from build123d import *

# Parameters (mm, degrees)
SKETCH1_R           = 5
BOSS_EXTRUDE1_DEPTH = 5


with BuildPart() as part:
    # Sketch1 → Boss-Extrude1 (new body)
    with BuildSketch(Plane.XY):
        Polygon((-56.800385751, 0), (-54.300385751, 0), (-54.300385751, -5), (-44.300385751, -5), (-44.300385751, 0), (-35.800385751, 0), (-35.800385751, 3), (-36.900385751, 3), (-36.900385751, 5.3), (-35.800385751, 5.3), (-35.800385751, 10), (-32.800385751, 10), (-32.800385751, 5.3), (-31.700385751, 5.3), (-31.700385751, 3), (-32.800385751, 3), (-32.800385751, 0), (-24.300385751, 0), (-24.300385751, -5), (-14.300385751, -5), (-14.300385751, -0.020707798), (-11.800385751, -0.020707798), (-11.800385751, 220), (-14.300385751, 220), (-14.300385751, 225), (-24.300385751, 225), (-24.300385751, 220), (-32.800385751, 220), (-32.800385751, 217), (-31.700385751, 217), (-31.700385751, 214.7), (-32.800385751, 214.7), (-32.800385751, 210), (-35.800385751, 210), (-35.800385751, 214.7), (-36.900385751, 214.7), (-36.900385751, 217), (-35.800385751, 217), (-35.800385751, 220), (-44.300385751, 220), (-44.300385751, 225), (-54.300385751, 225), (-54.300385751, 220), (-56.800385751, 220), align=None)
        with Locations((-44.300385751, 210)):
            Circle(SKETCH1_R, mode=Mode.SUBTRACT)
        with Locations((-24.300385751, 210)):
            Circle(SKETCH1_R, mode=Mode.SUBTRACT)
        with Locations((-24.300385751, 185)):
            Circle(SKETCH1_R, mode=Mode.SUBTRACT)
        with Locations((-24.300385751, 160)):
            Circle(SKETCH1_R, mode=Mode.SUBTRACT)
        with Locations((-24.300385751, 135)):
            Circle(SKETCH1_R, mode=Mode.SUBTRACT)
        with Locations((-24.300385751, 110)):
            Circle(SKETCH1_R, mode=Mode.SUBTRACT)
        with Locations((-24.300385751, 85)):
            Circle(SKETCH1_R, mode=Mode.SUBTRACT)
        with Locations((-24.300385751, 60)):
            Circle(SKETCH1_R, mode=Mode.SUBTRACT)
        with Locations((-24.300385751, 35)):
            Circle(SKETCH1_R, mode=Mode.SUBTRACT)
        with Locations((-24.300385751, 10)):
            Circle(SKETCH1_R, mode=Mode.SUBTRACT)
        with Locations((-44.300385751, 185)):
            Circle(SKETCH1_R, mode=Mode.SUBTRACT)
        with Locations((-44.300385751, 160)):
            Circle(SKETCH1_R, mode=Mode.SUBTRACT)
        with Locations((-44.300385751, 135)):
            Circle(SKETCH1_R, mode=Mode.SUBTRACT)
        with Locations((-44.300385751, 110)):
            Circle(SKETCH1_R, mode=Mode.SUBTRACT)
        with Locations((-44.300385751, 85)):
            Circle(SKETCH1_R, mode=Mode.SUBTRACT)
        with Locations((-44.300385751, 60)):
            Circle(SKETCH1_R, mode=Mode.SUBTRACT)
        with Locations((-44.300385751, 35)):
            Circle(SKETCH1_R, mode=Mode.SUBTRACT)
        with Locations((-44.300385751, 10)):
            Circle(SKETCH1_R, mode=Mode.SUBTRACT)
    extrude(amount=BOSS_EXTRUDE1_DEPTH)


solid = part.part
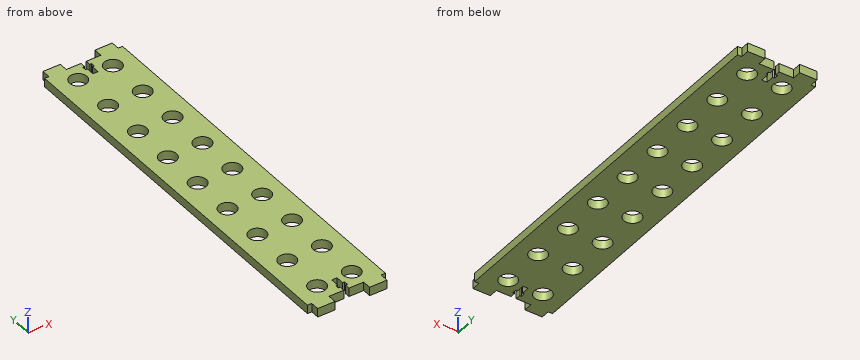
For this review, take the finished solid that the model builds, in its own axes (mm). Give positions to 0.01 mm unless a question says otherwise; leave off trailing zeros. Loops run counter-clockwise (first coordinate to the right, second up) from the corner with the lowest first, then second, coordinate; pieces in that order, holes last. Notation, with made-up numbers: M 57,-21.75 L 84,-21.75 A5 ccw 84,-16.75 Z; hole C -32.75,1 d9. An arc over 180 degrees is marked long. Answer as a JSON object with one key per item and string values. Group by question number.
Q1. Add section B-B on z = 2.1. Give the number of separate pieces and of enclosed holes in the cut face, and give its area (3 significant figures).
Q2. Add section C-C on y = 88. Give the boundary of the cut face in (x, z).
Q3. Add section A-A on y = 135. Give the boundary of the cut face in (x, z), and give its area (3 significant figures).
Q4. For probe 1 along Y at (x, z) = (-32, 0.7); probe 2 along X at (y, z) = (110.5, 3.7); probe 3 along X at (y, z) = (183.5, 2.45), list the stretches that pass through material, from the lowest coordinate up. Write a range as [from, to].
Q5. Insertion check: P1, Ø1.5, axis at x = -26.5, y = 39, coming from the +Z side; P2, Ø0.6, axis at x = -32.5, z = 2.5, coming from the +Y side; P3, Ø2, axis at x = -55.5, z = 2, coming from the -Y side; P4, Ø1.5, axis at y = -2.5, z = 3.5, coming from the -X side. Each pin has a flat end and moves straight along its axis. Give the tip position at first contact, or say it passes through.
Checked values:
{
 "1": {"separate pieces": "1", "enclosed holes": "18", "area": "8,620 mm²"},
 "2": {"outline": "M -56.8,0 L -48.3,0 L -48.3,5 L -56.8,5 Z; M -40.3,0 L -28.3,0 L -28.3,5 L -40.3,5 Z; M -20.3,0 L -11.8,0 L -11.8,5 L -20.3,5 Z"},
 "3": {"outline": "M -56.8,0 L -49.3,0 L -49.3,5 L -56.8,5 Z; M -39.3,0 L -29.3,0 L -29.3,5 L -39.3,5 Z; M -19.3,0 L -11.8,0 L -11.8,5 L -19.3,5 Z", "area": "125 mm²"},
 "4": {"probe 1": "[0, 3], [5.3, 214.7], [217, 220]", "probe 2": "[-56.8, -49.28], [-39.33, -29.28], [-19.33, -11.8]", "probe 3": "[-56.8, -49.07], [-39.53, -29.07], [-19.53, -11.8]"},
 "5": {"P1": "z = 5", "P2": "y = 220", "P3": "y = 0", "P4": "x = -54.3"}
}
